Read the model definition and answer for the solid it produces. Units are mm, in the model's axes. Give positions to 0.01 mm unless a question says otherwise; leave off trailing zeros. Write each loop counter-clockwise with the first axis right and the second up, starting at its lowest first coordinate (ties: lowest second). Pieces come first, ordered by that corner, then holes. Notation, with made-up numbers: M 37,-5.75 L 43,-5.75 A36 ccw 43,28.25 Z; hole C 8.25,13.25 d6. An arc over 180 degrees is marked long. Use a Markdown table: item, result. Add a question column.
Item 1: A cutting plane is placed at B-B on x = -321. Determine the outline of the cut face in (y, z), then the cut area to 3 significant figures.
Item 2: Given P1, Ø4, axis at y = -121.5, z = 7.5, coming from the -X side; P2, Ø5, axis at x = -327.5, z = 5.5, coming from the +Y side; P3, Ø3, axis at y = -166.5, z = 7, coming from the +X side, each flat-ended and moving along its own axis, determine where each tip first touches the part or whether it passes through.
Item 3: Consider probe 1 along Y at (x, z) = (-284, 8.75); probe 2 along Y at (x, z) = (-309.5, 5.5); probe 3 along Y at (x, z) = (-303, 5). Determine where each line is inside the solid, lowest interval first. Write a range as [from, to].
Item 4: A cutting plane is placed at C-C on y = -124. Determine the outline of the cut face in (x, z), then the cut area to 3 significant figures.
Item 5: A cutting plane is placed at A-A on z = 5. Count the separate pieces of the cut face and the enclosed holes in it, then the cut area to 3 significant figures.
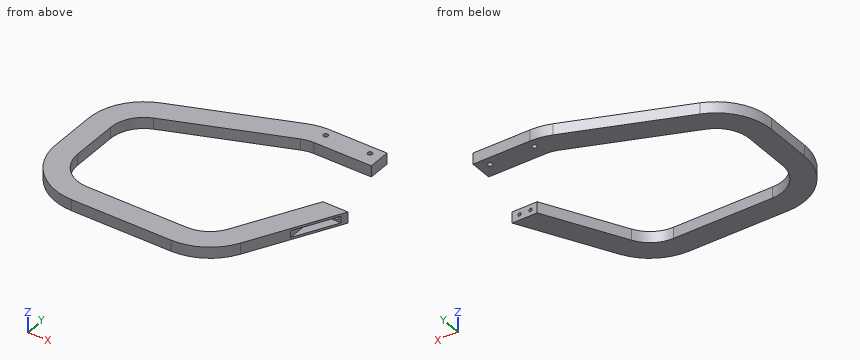
from build123d import *

# Parameters (mm, degrees)
SKETCH_1_R               = 2.1
EXTRUDE_1_DEPTH          = 10
CUT_EXTRUDE_1_DEPTH      = 3
CUT_EXTRUDE_1_DEPTH_BACK = 3
SKETCH_5_R               = 1.5
CUT_EXTRUDE_2_DEPTH      = 5


with BuildPart() as part:
    # 草图1 → 凸台-拉伸1 (new body)
    with BuildSketch(Plane.XY):
        with BuildLine():
            Line((-387.930073268, -240), (-298.601858772, -240))
            ThreePointArc((-298.601858772, -240), (-272.863892205, -232.866736253), (-254.469753791, -213.50228308))
            Line((-254.469753791, -213.50228308), (-212.930073268, -135.499923245))
            Line((-212.930073268, -135.499923245), (-235.589314209, -135.499923245))
            Line((-235.589314209, -135.499923245), (-272.122595783, -204.101369848))
            ThreePointArc((-272.122595783, -204.101369848), (-283.159078832, -215.720041752), (-298.601858772, -220))
            Line((-298.601858772, -220), (-387.930073268, -220))
            ThreePointArc((-387.930073268, -220), (-409.143276704, -211.213203436), (-417.930073268, -190))
            Line((-417.930073268, -190), (-417.930073268, -147.979949055))
            ThreePointArc((-417.930073268, -147.979949055), (-412.707094466, -131.065481267), (-398.856791899, -120.040607259))
            Line((-398.856791899, -120.040607259), (-295.350394851, -79.56058145))
            ThreePointArc((-295.350394851, -79.56058145), (-289.983341054, -78.019588665), (-284.42367622, -77.499923245))
            Line((-284.42367622, -77.499923245), (-232.930073268, -77.499923245))
            Line((-232.930073268, -77.499923245), (-232.930073268, -57.5))
            Line((-232.930073268, -57.5), (-284.423872481, -57.5))
            ThreePointArc((-284.423872481, -57.5), (-293.689980537, -58.366109034), (-302.635070198, -60.934430341))
            Line((-302.635070198, -60.934430341), (-406.141270986, -101.414379396))
            ThreePointArc((-406.141270986, -101.414379396), (-429.225108599, -119.789169409), (-437.930073268, -147.979949055))
            Line((-437.930073268, -147.979949055), (-437.930073268, -190))
            ThreePointArc((-437.930073268, -190), (-423.285412328, -225.355339059), (-387.930073268, -240))
        make_face()
        with Locations((-242.930073268, -65)):
            Circle(SKETCH_1_R, mode=Mode.SUBTRACT)
        with Locations((-282.930073268, -65)):
            Circle(SKETCH_1_R, mode=Mode.SUBTRACT)
    extrude(amount=EXTRUDE_1_DEPTH)

    # 草图4 → 切除-拉伸1 (cut, two sides: drawn at the far end of the back side and taken through both)
    with BuildSketch(Plane.XY.offset(5).offset(-CUT_EXTRUDE_1_DEPTH_BACK)):
        Polygon((-235.239731933, -167.152806322), (-235.239731933, -177.392542568), (-215.592792743, -140.499923245), (-230.589314209, -140.499923245), (-235.239731933, -140.499923245), align=None)
    extrude(amount=CUT_EXTRUDE_1_DEPTH + CUT_EXTRUDE_1_DEPTH_BACK, mode=Mode.SUBTRACT)

    # 草图5 → 切除-拉伸2 (cut)
    with BuildSketch(Plane.XZ.offset(140.499923245)):
        with Locations((-229.592792743, 5)):
            Circle(SKETCH_5_R)
        with Locations((-219.592792743, 5)):
            Circle(SKETCH_5_R)
    extrude(amount=-CUT_EXTRUDE_2_DEPTH, mode=Mode.SUBTRACT)


solid = part.part
Filled in:
| question | item | result |
|---|---|---|
| 1 | outline | M -240,0 L -220,0 L -220,10 L -240,10 Z; M -89.59,0 L -68.12,0 L -68.12,10 L -89.59,10 Z |
| 1 | area | 415 mm² |
| 2 | P1 | x = -431.53 |
| 2 | P2 | y = -69.68 |
| 2 | P3 | x = -228.84 |
| 3 | probe 1 | [-237.82, -216.21], [-77.5, -66.81], [-63.19, -57.5] |
| 3 | probe 2 | [-240, -220], [-85.09, -63.62] |
| 3 | probe 3 | [-240, -220], [-82.55, -61.08] |
| 4 | outline | M -431.8,0 L -405.96,0 L -405.96,10 L -431.8,10 Z |
| 4 | area | 258 mm² |
| 5 | separate pieces | 3 |
| 5 | enclosed holes | 2 |
| 5 | area | 10,500 mm² |
